from build123d import *


# Not quite as in the source:
# - a fillet or chamfer that OpenCascade refuses, or shapes differently, is made with other operations: its cross-section is extruded or revolved along the edge and cut away or added


with BuildPart() as f1:
    # F0 (on Right) → F1 (revolve)
    with BuildSketch(Plane.YZ):
        Polygon((-1.8, 0), (0, 0), (0, 8.2), (-1.8, 8.2), (-1.8, 6.2), (-1.4, 6.1908951029), (-1.4, 2), (-1.8, 2), align=None)
    revolve(axis=Axis((0, 0, 4.1), (0, 0, 1)))

    # F2: fillet of radius 1 on 2 edges, made by hand

    # F2_s1 → F2_t2 (revolve, cut)
    with BuildSketch(Plane.YZ):
        with BuildLine():
            ThreePointArc((-1.8, 6.9908951029), (-1.694427191, 6.5436815074), (-1.4, 6.1908951029))
            Line((-1.4, 6.1908951029), (-1.8, 6.2))
            Line((-1.8, 6.2), (-1.8, 6.9908951029))
        make_face()
    revolve(axis=Axis((0, 0, 6.2), (0, 0, 1)), mode=Mode.SUBTRACT)

    # F2_s3 → F2_t4 (revolve, cut)
    with BuildSketch(Plane.YZ):
        with BuildLine():
            ThreePointArc((-1.4, 2), (-1.694427191, 1.6472135955), (-1.8, 1.2))
            Line((-1.8, 1.2), (-1.8, 2))
            Line((-1.8, 2), (-1.4, 2))
        make_face()
    revolve(axis=Axis((0, 0, 2), (0, 0, 1)), mode=Mode.SUBTRACT)


solid = f1.part
Work out the finished part from the listing and answer in its coordinate system (mm). Coordinates: 2 decimals unless noted, no trailing zeros. Loops run counter-clockwise (first coordinate to the right, second up) from the corner with the lowest first, then second, coordinate; pieces in that order, holes last. Notation, with made-up numbers: M 84,65.5 L 104,65.5 A27 ccw 104,101.5 Z; hole C 17.5,-10.75 d4. An arc over 180 degrees is marked long. Answer in a Markdown table with one row per item. Add a question column.
1. The mould has two halves that part along Z. Classify faces 1 (the cylindrical face through (0.541, -1.717, 0.592)), 2 (the flat face through (0, 0, 8.2)), 3 (the cylindrical face through (0.06, 1.4, 4.07)): pulls with the +Z half, pulls with the -Z half, needs draft (parallel to the pull), parting line crosses it, or undercut.
2. Find section A-A, the plane z = 1. Write down the section's boundary in (x, y), then the cut area to 3 significant figures.
3. A flat-ended cylindrical pin translates along its axis: P1, Ø2, axis at y = -0.5, z = 4, coming from the +X side. Find the tip coordinate at first contact, or state that the pin passes through.
4. Consider L1, parallel to Z at x = -1.35, y = 1; L2, parallel to X at y = 0.05, z = 5.5; L3, parallel to Z at x = -0.6, y = 1.5. Determine where each line is inside the solid, lowest interval first.
5. Find section B-B, the plane z = 2.75. Write down the section's boundary in (x, y).
Reported:
| question | item | result |
|---|---|---|
| 1 | face 1 | needs draft |
| 1 | face 2 | pulls with the +Z half |
| 1 | face 3 | undercut |
| 2 | outline | C 0,0 d3.6 |
| 2 | area | 10.2 mm^2 |
| 3 | P1 | stops at x = 1.4 |
| 4 | L1 | z = 0 to 1.67, 6.52 to 8.2 |
| 4 | L2 | x = -1.4 to 1.4 |
| 4 | L3 | z = 0 to 1.78, 6.41 to 8.2 |
| 5 | outline | C 0,0 d2.8 |
